Source: CAD feature listing. Evaluate the final solid. Frame: model axes, mm. Face numbers are marked on the shaded views. A direction names the side the tool comes from. Give positions to 0.01 mm unless a question says otherwise; leave off trailing zeros. Order: outer loops, then holes, each group sorted by start corner. A loop starts at its lowest first (then second) coordinate and runs counter-clockwise, first axis right, second up.
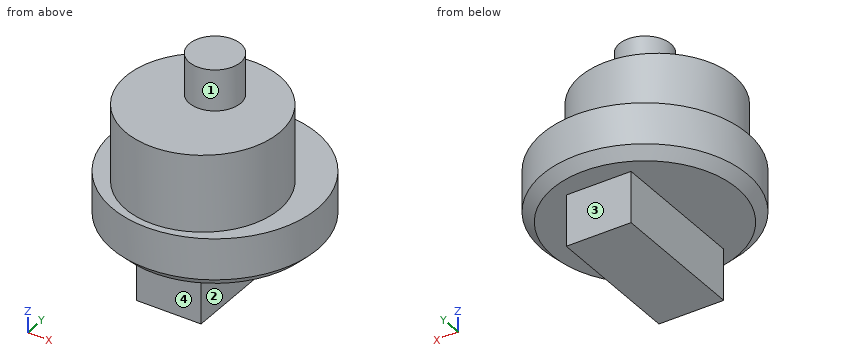
```python
from build123d import *

# Parameters (mm, degrees)
SKETCH1_R           = 10
BOSS_EXTRUDE1_DEPTH = 5
SKETCH2_R           = 7.5
BOSS_EXTRUDE2_DEPTH = 7.5
SKETCH3_R           = 2.5
BOSS_EXTRUDE3_DEPTH = 4
SKETCH4_W           = 6.306649828
SKETCH4_H           = 13.679653114
BOSS_EXTRUDE4_DEPTH = 5
CHAMFER2_SIZE       = 1


with BuildPart() as part:
    # Sketch1 → Boss-Extrude1 (new body)
    with BuildSketch(Plane.XY):
        Circle(SKETCH1_R)
    extrude(amount=BOSS_EXTRUDE1_DEPTH)

    # Sketch2 → Boss-Extrude2 (add)
    with BuildSketch(Plane.XY.offset(5)):
        with Locations((0, -1.812)):
            Circle(SKETCH2_R)
    extrude(amount=BOSS_EXTRUDE2_DEPTH)

    # Sketch3 → Boss-Extrude3 (add)
    with BuildSketch(Plane.XY.offset(12.5)):
        Circle(SKETCH3_R)
    extrude(amount=BOSS_EXTRUDE3_DEPTH)

    # Sketch4 → Boss-Extrude4 (add)
    with BuildSketch(Plane(origin=(0, 0, 0), x_dir=(-1, 0, 0), z_dir=(0, 0, -1))):
        Rectangle(SKETCH4_W, SKETCH4_H)
    extrude(amount=BOSS_EXTRUDE4_DEPTH)

    # Chamfer2
    chamfer2_edges = [part.edges().sort_by_distance(p)[0] for p in [
        (-10, 0, 0),
    ]]
    chamfer(chamfer2_edges, length=CHAMFER2_SIZE)


solid = part.part
```
1) Material intervals for L1, parallel to Z at x = -5.25, y = 5; L2, parallel to Z at x = 0.5, y = -5; L3, parallel to X at y = 1.5, z = -2.75, sorted ascending.
Report:
L1: z = 0 to 5
L2: z = -5 to 12.5
L3: x = -3.15 to 3.15
2) Section query B-B, the plane y = 0. Return the cut outline in (x, z), and give its area (3 significant figures).
Report:
outline: (-10, 1) - (-9, 0) - (-3.15, 0) - (-3.15, -5) - (3.15, -5) - (3.15, 0) - (9, 0) - (10, 1) - (10, 5) - (7.28, 5) - (7.28, 12.5) - (2.5, 12.5) - (2.5, 16.5) - (-2.5, 16.5) - (-2.5, 12.5) - (-7.28, 12.5) - (-7.28, 5) - (-10, 5) - close
area: 260 mm2
3) Pin query (flat end, axial travel): pin 1 (5 mm diameter, centred on y = 4.5, z = -1.5, fed in from -X); pin 2 (2.5 mm diameter, centred on x = -1, z = -2.5, fed in from +Y); pin 3 (5 mm diameter, centred on x = 6.5, y = -5, fed in from -Z). Return the tip coordinate at first contact, or that it passes through.
Report:
pin 1: stops at x = -9.15
pin 2: stops at y = 6.84
pin 3: stops at z = 0
4) Section query A-A, the plane x = 0. Return the cut outline in (y, z), and give its area (3 significant figures).
Report:
outline: (-10, 1) - (-9, 0) - (-6.84, 0) - (-6.84, -5) - (6.84, -5) - (6.84, 0) - (9, 0) - (10, 1) - (10, 5) - (5.69, 5) - (5.69, 12.5) - (2.5, 12.5) - (2.5, 16.5) - (-2.5, 16.5) - (-2.5, 12.5) - (-9.31, 12.5) - (-9.31, 5) - (-10, 5) - close
area: 300 mm2
5) Reachability of the marked faces 1, 2, 3 and 4 from +Z, -Z, +X, -X, +Y, -Y: full face, straight path, thin tool, end or side. Return the list, or none.
Report:
face 1: +Z
face 2: -Z, +X, +Y, -Y
face 3: -Z, +X, -X, +Y
face 4: -Z, +X, -X, -Y
6) Section query D-D, the plane z = 4. Return the cut outline in (x, y), and give its area (3 significant figures).
Report:
outline: circle Ø20 at (0, 0)
area: 314 mm2
7) Section query C-C, the plane z = 15. Return the cut outline in (x, y), and give its area (3 significant figures).
Report:
outline: circle Ø5 at (0, 0)
area: 19.6 mm2
